Build history of the part. All positions in model axes, mm. Face numbers are marked on the shaded views. A direction names the side the tool comes from. Give positions to 0.01 mm unless a question says otherwise; leave off trailing zeros. Order: outer loops, then holes, each group sorted by start corner. A loop starts at its lowest first (then second) coordinate and runs counter-clockwise, first axis right, second up. Notation, with made-up numbers: M 20.5,-36.5 L 77.5,-36.5 A31 ccw 77.5,-8.5 Z; hole C 23.5,53 d11. An arc over 180 degrees is marked long. One line per item, written item: value. Start each with the question number.
from build123d import *

# Parameters (mm, degrees)
SKETCH1_R           = 38.1
SKETCH1_R_2         = 1.5875
BOSS_EXTRUDE1_DEPTH = 2.54
SKETCH2_R           = 1.5875
BOSS_EXTRUDE2_DEPTH = 28.956
SKETCH3_W           = 26.67
SKETCH3_H           = 17.78
CUT_EXTRUDE1_DEPTH  = 45.72


with BuildPart() as part:
    # Sketch1 → Boss-Extrude1 (new body)
    with BuildSketch(Plane(origin=(0, 0, 0), x_dir=(1, 0, 0), z_dir=(0, 1, 0))):
        with Locations(Location((0, 0, 0), (0, 0, 270))):
            Circle(SKETCH1_R)
        with Locations(Location((0, 29.337, 0), (0, 0, 270))):
            Circle(SKETCH1_R_2, mode=Mode.SUBTRACT)
        with Locations(Location((25.406587271, -14.6685, 0), (0, 0, 270))):
            Circle(SKETCH1_R_2, mode=Mode.SUBTRACT)
        with Locations(Location((-25.406587271, -14.6685, 0), (0, 0, 270))):
            Circle(SKETCH1_R_2, mode=Mode.SUBTRACT)
    extrude(amount=BOSS_EXTRUDE1_DEPTH)


with BuildPart() as body_2:
    # Sketch2 → Boss-Extrude2 (new body)
    with BuildSketch(Plane(origin=(0, 2.54, 0), x_dir=(1, 0, 0), z_dir=(0, 1, 0))):
        with BuildLine():
            Line((25.406587271, -11.176), (18.270749664, 25.342499299))
            Line((18.270749664, 25.342499299), (3.4925, 29.337))
            ThreePointArc((3.4925, 29.337), (0, 32.8295), (-3.4925, 29.337))
            Line((-3.4925, 29.337), (-18.270749664, 25.342499299))
            Line((-18.270749664, 25.342499299), (-25.406587271, -11.176))
            ThreePointArc((-25.406587271, -11.176), (-28.899087271, -14.6685), (-25.406587271, -18.161))
            Line((-25.406587271, -18.161), (-21.295139445, -22.86))
            Line((-21.295139445, -22.86), (21.295139445, -22.86))
            Line((21.295139445, -22.86), (25.406587271, -18.161))
            ThreePointArc((25.406587271, -18.161), (28.899087271, -14.6685), (25.406587271, -11.176))
        make_face()
        with Locations(Location((25.406587271, -14.6685, 0), (0, 0, 270))):
            Circle(SKETCH2_R, mode=Mode.SUBTRACT)
        with Locations(Location((0, 29.337, 0), (0, 0, 270))):
            Circle(SKETCH2_R, mode=Mode.SUBTRACT)
        with Locations(Location((-25.406587271, -14.6685, 0), (0, 0, 270))):
            Circle(SKETCH2_R, mode=Mode.SUBTRACT)
    extrude(amount=BOSS_EXTRUDE2_DEPTH)

    # Sketch3 → Cut-Extrude1 (cut)
    with BuildSketch(Plane.XY.offset(22.86)):
        with Locations((0, 27.178)):
            Rectangle(SKETCH3_W, SKETCH3_H)
        with Locations((0, 6.858)):
            Rectangle(SKETCH3_W, SKETCH3_H)
    extrude(amount=-CUT_EXTRUDE1_DEPTH, mode=Mode.SUBTRACT)


solid = body_2.part
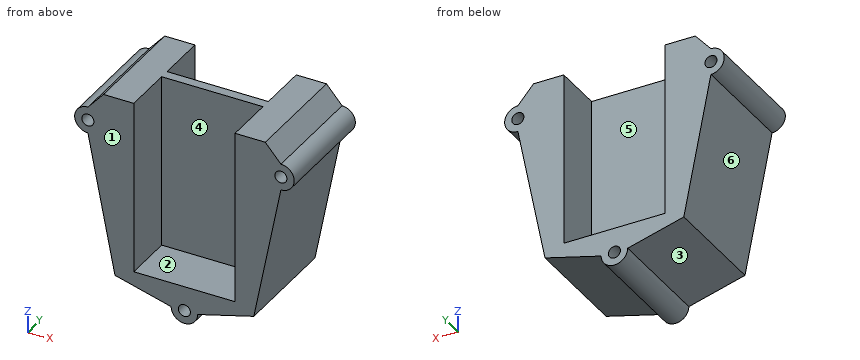
1) Slice it at C-C (z = -10.5). List the corners of the cut face in (x, y) (3 decimals).
2) Slice it at B-B (y = 20.25). List the corners of the cut face in (x, z) (1 decimal), plus the area to 3 significant figures.
3) Drop flat-ended pins along their axis: P1, Ø4, axis at x = 25.41, z = 14.67, coming from the -Y side; P2, Ø2, axis at y = 13, z = 4, coming from the +X side; P3, Ø6.5, axis at y = 12.5, z = 3.5, coming from the +X side; P4, Ø10.5, axis at y = 27, z = 4, coming from the +X side. Give the stop position or say it passes through.
4) Tool access for the marked faces 4, 5 and 6: list every direction of +Z, -Z, +X, -X, +Y, -Y with a clear straight run to the whole face (end or side of a thin tool).
5) Pull direction X, two halves, no side cores. Call the marked faces 1, 2 and 3: pulls with the +X half, pulls with the -X half, needs draft (parallel to the pull), parting line crosses it, or undercut.
6) Drill centre lines: line 1 (Z direction, x = -25.5, y = 20.5); line 2 (X direction, y = 21.75, z = 8) (3 decimals); line 3 (X direction, y = 6.5, z = -29.5). Where is each one in solid material? Low to high.
7) Slice it at D-D (x = -10.5). List the corners of the cut face in (y, z).
8) Slice it at A-A (x = 0). List the corners of the cut face in (y, z), plus the area to 3 significant figures.
Results list:
1. outline: M -21.171,2.54 L -13.335,2.54 L -13.335,15.748 L 13.335,15.748 L 13.335,2.54 L 21.171,2.54 L 21.171,31.496 L 13.335,31.496 L 13.335,18.288 L -13.335,18.288 L -13.335,31.496 L -21.171,31.496 Z
2. outline: M -25.4,11.2 L -18.3,-25.3 L -3.5,-29.3 A3.5 ccw 3.5,-29.3 L 18.3,-25.3 L 25.4,11.2 A3.5 ccw 25.4,18.2 L 21.3,22.9 L 13.3,22.9 L 13.3,-22.9 L -13.3,-22.9 L -13.3,22.9 L -21.3,22.9 L -25.4,18.2 A3.5 ccw Z; hole C -25.4,14.7 d3.2; hole C 0,-29.3 d3.2; hole C 25.4,14.7 d3.2
2. area: 1,070 mm²
3. P1: stops at y = 2.54
3. P2: stops at x = 24.2
3. P3: stops at x = 24.54
3. P4: stops at x = 25.03
4. face 4: +Z, -Y
4. face 5: +Z, +Y
4. face 6: -Z, -X, +Y, -Y
5. face 1: needs draft
5. face 2: undercut
5. face 3: pulls with the -X half
6. line 1: z = 11.18 to 13.08, 16.25 to 18.16
6. line 2: x = -24.786 to -13.335, 13.335 to 24.786
6. line 3: x = -3.49 to -1.58, 1.58 to 3.49
7. outline: M 2.54,-27.44 L 31.5,-27.44 L 31.5,-22.86 L 18.29,-22.86 L 18.29,22.86 L 15.75,22.86 L 15.75,-22.86 L 2.54,-22.86 Z
8. outline: M 2.54,-32.83 L 31.5,-32.83 L 31.5,-30.92 L 2.54,-30.92 Z; M 2.54,-27.75 L 31.5,-27.75 L 31.5,-22.86 L 18.29,-22.86 L 18.29,22.86 L 15.75,22.86 L 15.75,-22.86 L 2.54,-22.86 Z
8. area: 313 mm²
